from build123d import *

# Parameters (mm, degrees)
BODY_DEPTH      = 10.2
SKETCH_2_R      = 2.5
SCREWHOLE_DEPTH = 10.2
CHAMFER_2_SIZE  = 0.2
FILLET_2_R      = 0.2


with BuildPart() as part:
    # Эскиз1 → Body (new body)
    with BuildSketch(Plane(origin=(0, 0, 0), x_dir=(0, 0, -1), z_dir=(1, 0, 0))):
        Polygon((-2.9, 0), (2.9, 0), (4.7, 1.5), (4.7, 3), (2.9, 3), (2.9, 4.5), (-2.9, 4.5), (-2.9, 3), (-4.7, 3), (-4.7, 1.5), align=None)
    extrude(amount=BODY_DEPTH)

    # Эскиз2 → screwHole (cut)
    with BuildSketch(Plane(origin=(0, 4.5, 0), x_dir=(1, 0, 0), z_dir=(0, 1, 0))):
        with Locations((5.1, 0)):
            Circle(SKETCH_2_R)
    extrude(amount=-SCREWHOLE_DEPTH, mode=Mode.SUBTRACT)

    # Chamfer 2
    chamfer_2_edges = [part.edges().sort_by_distance(p)[0] for p in [
        (2.6, 4.5, 0),
    ]]
    chamfer(chamfer_2_edges, length=CHAMFER_2_SIZE)

    # Fillet 2
    fillet_2_edges = [part.edges().sort_by_distance(p)[0] for p in [
        (5.1, 3, 4.7),
        (5.1, 3, -4.7),
    ]]
    fillet(fillet_2_edges, radius=FILLET_2_R)


solid = part.part
For this review, take the finished solid that the model builds, in its own axes (mm). A direction names the side the tool comes from. Coordinates: 2 decimals unless noted, no trailing zeros. Loops run counter-clockwise (first coordinate to the right, second up) from the corner with the lowest first, then second, coordinate; pieces in that order, holes last. Notation, with made-up numbers: (52, 19) - (108, 19) arc R28 ccw to (108, 48) - close; hole circle Ø8 at (76.25, -19.75). An arc over 180 degrees is marked (long way). Return JSON: item names as keys, results as strings.
Item 1: For faces 5 (the flat face through (5, 4, -2.9)), 6 (the flat face through (2.76, 0, -1.25)), 7 (the flat face through (5, 4, 2.9)), list the 3-axis set-ups (+Z, -Z, +X, -X, +Y, -Y) from which the entire face can be reached by the end or side of a thin tool; tool diameter is ignored.
Determined:
{"face 5": "-Z, +X, -X, +Y", "face 6": "+Z, -Z, +X, -X, -Y", "face 7": "+Z, +X, -X, +Y"}
Item 2: Mouldability with a two-part tool opening along X and no side actions: class faces 1 (the flat face through (0, 2, 0)), 2 (the flat face through (5.03, 0.74, -3.79)), 3 (the flat face through (10.2, 2, 0)), 4 (the cylindrical face through (3.1, 2.2, 1.5)) as pulls with the +X half, pulls with the -X half, needs draft (parallel to the pull), parting line crosses it, or undercut.
Determined:
{"face 1": "pulls with the -X half", "face 2": "needs draft", "face 3": "pulls with the +X half", "face 4": "undercut"}
Item 3: For line 1 (X direction, y = 1.05, z = 0); line 2 (Z direction, x = 5.1, y = 1.95); line 3 (X direction, y = 2.8, z = -0.5), list the stretches that pass through material, from the lowest coordinate up.
Determined:
{"line 1": "x = 0 to 2.6, 7.6 to 10.2", "line 2": "z = -4.7 to -2.5, 2.5 to 4.7", "line 3": "x = 0 to 2.65, 7.55 to 10.2"}
Item 4: Take a section at A-A (z = 0). Give the boundary of the cut face in (x, y), then the cut area to 3 significant figures.
Determined:
{"outline": "(0, 0) - (2.6, 0) - (2.6, 4.3) - (2.4, 4.5) - (0, 4.5) - close; (7.6, 0) - (10.2, 0) - (10.2, 4.5) - (7.8, 4.5) - (7.6, 4.3) - close", "area": "23.4 mm2"}
Item 5: Take a section at C-C (x = 5.1). Give the boundary of the cut face in (y, z), then the cut area to 3 significant figures.
Determined:
{"outline": "(0, -2.9) - (1.5, -4.7) - (2.8, -4.7) arc R0.2 ccw to (3, -4.5) - (3, -2.9) - (4.5, -2.9) - (4.5, -2.7) - (4.3, -2.5) - (0, -2.5) - close; (0, 2.5) - (4.3, 2.5) - (4.5, 2.7) - (4.5, 2.9) - (3, 2.9) - (3, 4.5) arc R0.2 ccw to (2.8, 4.7) - (1.5, 4.7) - (0, 2.9) - close", "area": "11.6 mm2"}
Item 6: Insertion check: pin 1 (0.5 mm diameter, centred on x = 7.5, z = 3.5, fed in from +Y); pin 2 (1.6 mm diameter, centred on x = 6, y = 4, fed in from +Z). Each pin has a flat end and moves straight along its axis. Give the tip position at first contact, or say it passes through.
Determined:
{"pin 1": "stops at y = 3", "pin 2": "stops at z = 2.9"}
Item 7: Take a section at D-D (x = 1.5). Give the boundary of the cut face in (y, z).
Determined:
{"outline": "(0, -2.9) - (1.5, -4.7) - (2.8, -4.7) arc R0.2 ccw to (3, -4.5) - (3, -2.9) - (4.5, -2.9) - (4.5, 2.9) - (3, 2.9) - (3, 4.5) arc R0.2 ccw to (2.8, 4.7) - (1.5, 4.7) - (0, 2.9) - close"}
Item 8: Take a section at B-B (y = 2.4). Give the boundary of the cut face in (x, z).
Determined:
{"outline": "(0, -4.7) - (10.2, -4.7) - (10.2, 4.7) - (0, 4.7) - close; hole circle Ø5 at (5.1, 0)"}
